Can you work these out from the model? Positions are in its coordinate system, mm. A direction names the side the tool comes from. Coordinates: 2 decimals unless noted, no trailing zeros. Loops run counter-clockwise (first coordinate to the right, second up) from the corner with the lowest first, then second, coordinate; pieces in that order, holes last.
```python
from build123d import *

# Parameters (mm, degrees)
RESSALTO_EXTRUS_O6_DEPTH   = 15
CORTE_EXTRUS_O1_DEPTH      = 46.47737596
CORTE_EXTRUS_O1_DEPTH_BACK = 46.47737596
ESBO_O14_R                 = 1.75
ESBO_O15_R                 = 1.75
CORTE_EXTRUS_O2_DEPTH      = 35.802205001
ESBO_O17_W                 = 10
ESBO_O17_H                 = 15
RESSALTO_EXTRUS_O7_DEPTH   = 2
FILETE1_R                  = 10


with BuildPart() as part:
    # Esboço13 → Ressalto-extrusão6 (new body)
    with BuildSketch(Plane(origin=(0, 0, 0), x_dir=(1, 0, 0), z_dir=(0, 1, 0))):
        with BuildLine():
            Line((-2.8, 15), (0, 15))
            Line((0, 15), (0, 15.348469228))
            Line((0, 15.348469228), (0, 16.348469228))
            Line((0, 16.348469228), (0, 18))
            Line((0, 18), (-8, 18))
            Line((-8, 18), (-8, 12.093386622))
            ThreePointArc((-8, 12.093386622), (-14.496982121, -0.295819827), (-7.5, -12.409673646))
            Line((-7.5, -12.409673646), (-7.5, -22.409673646))
            Line((-7.5, -22.409673646), (-5, -22.409673646))
            Line((-5, -22.409673646), (-5, -10.908712115))
            ThreePointArc((-5, -10.908712115), (-11.943432553, 1.16379502), (-2.8, 11.668761717))
            Line((-2.8, 11.668761717), (-2.8, 15))
        make_face()
        with BuildLine():
            ThreePointArc((2.8, 11.668761717), (11.943432553, 1.16379502), (5, -10.908712115))
            Line((5, -10.908712115), (5, -22.409673646))
            Line((5, -22.409673646), (7.5, -22.409673646))
            Line((7.5, -22.409673646), (7.5, -12.409673646))
            ThreePointArc((7.5, -12.409673646), (14.496982121, -0.295819827), (8, 12.093386622))
            Line((8, 12.093386622), (8, 18))
            Line((8, 18), (0, 18))
            Line((0, 18), (0, 16.348469228))
            Line((0, 16.348469228), (0, 15.348469228))
            Line((0, 15.348469228), (0, 15))
            Line((0, 15), (2.8, 15))
            Line((2.8, 15), (2.8, 11.668761717))
        make_face()
    extrude(amount=RESSALTO_EXTRUS_O6_DEPTH)

    # Esboço14 → Corte-extrusão1 (cut, two sides: drawn at the far end of the back side and taken through both)
    with BuildSketch(Plane(origin=(0, 0, -18), x_dir=(-1, 0, 0), z_dir=(0, 0, -1)).offset(-CORTE_EXTRUS_O1_DEPTH_BACK)):
        with Locations((0, 12.5)):
            Circle(ESBO_O14_R)
        with Locations((0, 2.5)):
            Circle(ESBO_O14_R)
    extrude(amount=CORTE_EXTRUS_O1_DEPTH + CORTE_EXTRUS_O1_DEPTH_BACK, mode=Mode.SUBTRACT)

    # Esboço15 → Corte-extrusão2 (cut, through all)
    with BuildSketch(Plane(origin=(7.5, 0, 0), x_dir=(0, 0, -1), z_dir=(1, 0, 0))):
        with Locations((-17.409673646, 7.5)):
            Circle(ESBO_O15_R)
    extrude(amount=-CORTE_EXTRUS_O2_DEPTH, mode=Mode.SUBTRACT)

    # Esboço17 → Ressalto-extrusão7 (add)
    with BuildSketch(Plane(origin=(7.5, 0, 0), x_dir=(0, 0, -1), z_dir=(1, 0, 0))):
        with Locations((-17.409673646, 7.5)):
            Rectangle(ESBO_O17_W, ESBO_O17_H)
        Polygon((-17.409673646, 10.733161507), (-20.209673646, 9.116580754), (-20.209673646, 5.883419246), (-17.409673646, 4.266838493), (-14.609673646, 5.883419246), (-14.609673646, 9.116580754), align=None, mode=Mode.SUBTRACT)
    extrude(amount=RESSALTO_EXTRUS_O7_DEPTH)

    # Filete1
    # the kernel refuses this fillet: 10 mm, written as the material it adds along each edge
    with BuildSketch(Plane(origin=(7.5, 0, 12.409673646), x_dir=(0.7539844158894258, 0, -0.656892305173292), z_dir=(0, 1, 0))) as filete1_piece_1:
        with BuildLine():
            CenterArc((6.715896851, -9.850615741), FILETE1_R, 99.91590085, 21.469545267)
            Line((1.507968832, -1.31378461), (0, 0))
            ThreePointArc((0, 0), (2.496936009, -0.216607176), (4.993872017, 0))
        make_face()
    extrude(amount=15)


solid = part.part
```
(1) Which directions (+Z, -Z, +X, -X, +Y, -Y) give clear straight access to the entire face, cutting with the end or side of a thin tool? Please do faces 4 (the flat face through (8, 8, 20.21)), 5 (the flat face through (8, 7, -15)), 6 (the flat face through (12, 0, 3)), 7 (the flat face through (9.5, 8, 14)), 8 (the cylindrical face through (-11.96, 7.4, -0.96)).
Check values:
face 4: +X
face 5: -Z, +X, +Y, -Y
face 6: +Z, -Z, +X, -X, -Y
face 7: +Z, +X, +Y, -Y
face 8: +Y, -Y
(2) I want a section at B-B on z = 14. Write out the boundary of the cut face in (x, y).
Check values:
outline: (-7.5, 0) - (-5, 0) - (-5, 15) - (-7.5, 15) - close; (5, 0) - (9.5, 0) - (9.5, 15) - (5, 15) - close
(3) If we mould it in two halves opening along X, with no side actions, what happens to faces 1 (the cylindrical face through (11.92, 7.4, -1.37)), 2 (the flat face through (8, 7, 14.61)), 3 (the flat face through (-8, 7, -15))? For each: released by +X, released by -X, zero draft, split by the parting line, or undercut.
Check values:
face 1: undercut
face 2: zero draft
face 3: released by -X
(4) I'm going to push flat-ended pins straight in: pin 1 (3 mm diameter, centred on y = 6.5, z = 17, fed in from +X); pin 2 (3.5 mm diameter, centred on y = 7, z = 19, fed in from -X); pin 3 (5.5 mm diameter, centred on x = 0, y = 2.5, fed in from +Z). Where does each tip first touch, or does it pass through?
Check values:
pin 1: stops at x = 7.5
pin 2: stops at x = -7.5
pin 3: stops at z = -15
(5) I want a section at A-A on y = 7.5. State how many separate pieces and enclosed holes the cut face has, then the cut area to 3 significant figures.
Check values:
separate pieces: 3
enclosed holes: 0
area: 274 mm2
(6) I want a section at D-D on y = 2.5. Write out the boundary of the cut face in (x, z), then the cut area to 3 significant figures.
Check values:
outline: (-8, -18) - (-1.75, -18) - (-1.75, -15) - (-2.8, -15) - (-2.8, -11.67) arc R12 cw to (-5, 10.91) - (-5, 22.41) - (-7.5, 22.41) - (-7.5, 12.41) arc R14.5 ccw to (-8, -12.09) - close; (1.75, -18) - (8, -18) - (8, -12.09) arc R14.5 ccw to (11.27, 9.13) arc R10 cw to (9.5, 12.41) - (9.5, 22.41) - (5, 22.41) - (5, 10.91) arc R12 cw to (2.8, -11.67) - (2.8, -15) - (1.75, -15) - close
area: 292 mm2
(7) I want a section at C-C on x = 0. Write out the boundary of the cut face in (y, z), then the cut area to 3 significant figures.
Check values:
outline: (0, -18) - (0.75, -18) - (0.75, -15) - (0, -15) - close; (4.25, -18) - (10.75, -18) - (10.75, -15) - (4.25, -15) - close; (14.25, -18) - (15, -18) - (15, -15) - (14.25, -15) - close
area: 24.0 mm2
(8) If I drill on probe 1 along Y at (x, z) = (0, -16.75); probe 2 along X at (y, z) = (1.5, 13); probe 3 along X at (y, z) = (5.75, 16.5), over which ranges is the centre line in solid material (lowest first)?
Check values:
probe 1: y = 0 to 0.75, 4.25 to 10.75, 14.25 to 15
probe 2: x = -7.5 to -5, 5 to 9.5
probe 3: x = -7.5 to -5, 5 to 7.5
